```python
from build123d import *

# Parameters (mm, degrees)
SKETCH1_W           = 22
SKETCH1_H           = 28
BOSS_EXTRUDE1_DEPTH = 1.6
SKETCH2_W           = 6
SKETCH2_H           = 6
BOSS_EXTRUDE2_DEPTH = 4
SKETCH3_W           = 12.5
SKETCH3_H           = 5.7
SKETCH3_W_2         = 7.5
BOSS_EXTRUDE3_DEPTH = 7
SKETCH5_R           = 1.55
SKETCH6_R           = 1.75


with BuildPart() as part:
    # Sketch1 → Boss-Extrude1 (new body)
    with BuildSketch(Plane.XY):
        with Locations((0, 14)):
            Rectangle(SKETCH1_W, SKETCH1_H)
    extrude(amount=BOSS_EXTRUDE1_DEPTH)

    # Sketch2 → Boss-Extrude2 (add)
    with BuildSketch(Plane.XY.offset(1.6)):
        with Locations((7.25, 22.75)):
            Rectangle(SKETCH2_W, SKETCH2_H)
    boss_extrude2 = extrude(amount=BOSS_EXTRUDE2_DEPTH)

    # Sketch3 → Boss-Extrude3 (add)
    with BuildSketch(Plane(origin=(0, 0, 0), x_dir=(-1, 0, 0), z_dir=(0, 0, -1))):
        with Locations((-4.25, 9.85)):
            Rectangle(SKETCH3_W, SKETCH3_H)
        with Locations((6.75, 9.85)):
            Rectangle(SKETCH3_W_2, SKETCH3_H)
    extrude(amount=BOSS_EXTRUDE3_DEPTH)

    # Sketch5 → Loft1 section 0
    with BuildSketch(Plane.XY.offset(11.6)):
        with Locations((7.25, 22.75)):
            Circle(SKETCH5_R)
    # Sketch6 → Loft1 section 1
    with BuildSketch(Plane.XY.offset(5.6)):
        with Locations((7.25, 22.75)):
            Circle(SKETCH6_R)
    loft1 = loft()

    # Mirror1: Boss-Extrude2, Loft1 across plane
    add(boss_extrude2.mirror(Plane(origin=(0, 0, 0), x_dir=(0, 0, 1), z_dir=(1, 0, 0))))
    add(loft1.mirror(Plane(origin=(0, 0, 0), x_dir=(0, 0, 1), z_dir=(1, 0, 0))))


solid = part.part
```
Part model, mm, in its own coordinate system. A direction names the side the tool comes from. Coordinates: 2 decimals unless noted, no trailing zeros. Order: outer loops, then holes, each group sorted by start corner. A loop starts at its lowest first (then second) coordinate and runs counter-clockwise, first axis right, second up. Notation, with made-up numbers: (16, 87) -> (41, 87) arc R20 ccw to (41, 108) -> close; hole circle Ø10 at (-12.5, -20). An arc over 180 degrees is marked (long way). Put each result on its own line as item: value. Start each with the question number.
(1) Band-saw the part on B-B (y = 11.75). Give the cut face in (x, z), then the cut area to 3 significant figures.
(2) Probe line 1 along X through (y, z) = (11.25, -1.5); line 2 along Y through (x, z) = (-6, -1.25); line 3 along Z through (x, y) = (0.25, 12.5). List the from-to ranges inside material, lowest first. Write a range as [from, to].
(3) Mould opens along X. For faces 5 (the face through (-10.25, 23, 4)), 6 (the face through (10.5, 10, -3)), 7 (the face through (-4.25, 23, 4)) say: pulls with the +X half, pulls with the -X half, needs draft (parallel to the pull), parting line crosses it, or undercut.
(4) Band-saw the part on D-D (y = 4.75). Give the cut face in (x, z).
(5) Band-saw the part on A-A (x = 7.25). Give the cut face in (y, z), then the cut area to 4 significant figures.
(6) Pin check, flat tips, straight feed: pin 1 Ø2 at (y, z) = (22, 2.5) entering from +X; pin 2 Ø1 at (x, y) = (0, 12.5) entering from +Z; pin 3 Ø1 at (y, z) = (11.5, -4.5) entering from -X; pin 4 Ø2 at (y, z) = (22, 3.5) entering from -X. Stop position of each tip, or through.
(7) Which spindle directions (+Z, -Z, +X, -X, +Y, -Y) get a long thin tool onto all of the face, cutting with end or side? Do faces 1 (the face through (-2, 10, -3)), 2 (the face through (-7, 12.7, -3)), 3 (the face through (4.25, 23, 4)), 4 (the face through (-6, 21, 5.6)). Say none if no direction does.
(8) Band-saw the part on C-C (x = 2). Give the cut face in (y, z), then the cut area to 3 significant figures.
Determined:
1. outline: (-11, 0) -> (-10.5, 0) -> (-10.5, -7) -> (-3, -7) -> (-3, 0) -> (-2, 0) -> (-2, -7) -> (10.5, -7) -> (10.5, 0) -> (11, 0) -> (11, 1.6) -> (-11, 1.6) -> close
1. area: 175 mm²
2. line 1: x = [-10.5, -3], [-2, 10.5]
2. line 2: y = [7, 12.7]
2. line 3: z = [-7, 1.6]
3. face 5: pulls with the -X half
3. face 6: pulls with the +X half
3. face 7: undercut
4. outline: (-11, 0) -> (11, 0) -> (11, 1.6) -> (-11, 1.6) -> close
5. outline: (0, 0) -> (7, 0) -> (7, -7) -> (12.7, -7) -> (12.7, 0) -> (28, 0) -> (28, 1.6) -> (25.75, 1.6) -> (25.75, 5.6) -> (24.5, 5.6) -> (24.3, 11.6) -> (21.2, 11.6) -> (21, 5.6) -> (19.75, 5.6) -> (19.75, 1.6) -> (0, 1.6) -> close
5. area: 128.5 mm²
6. pin 1: stops at x = 11
6. pin 2: stops at z = 1.6
6. pin 3: stops at x = -10.5
6. pin 4: stops at x = -10.25
7. face 1: -Z, +Y, -Y
7. face 2: -Z, +X, -X, +Y
7. face 3: +Z, +Y, -Y
7. face 4: +Z
8. outline: (0, 0) -> (7, 0) -> (7, -7) -> (12.7, -7) -> (12.7, 0) -> (28, 0) -> (28, 1.6) -> (0, 1.6) -> close
8. area: 84.7 mm²
